The figure shows three views and two pictorial views of one solid part (mm, origin at its lowest corner). Answer the questions. Give positions to 0.01 mm unless a question says otherwise; leave off trailing zeros. Write each loop counter-clockwise with the first axis right and the second up, starting at its lowest first coordinate (ties: lowest second). Pieces come first, ordered by that corner, then holes. Notation, with made-up numbers: (-28, 89.5) - (14, 89.5) arc R8 ccw to (14, 104.5) - close; hole circle Ø8 at (76.5, -20.75). An arc over 180 degrees is marked (long way). Answer as CSV lines item,"result". Start each with the question number.
(1) Find section C-C (x = 269). Write down the section's boundary in (y, z).
(2) Find section B-B (y = 28). Write down the section's boundary in (x, z).
(3) Straight lines are drawn through the part: probe 1 along X at (y, z) = (12, 369); probe 2 along Z at (x, y) = (543, 39). For each, find the intervals that lie inside material, in ascending order.
(4) Find section A-A (z = 620.5). Write down the section's boundary in (x, y).
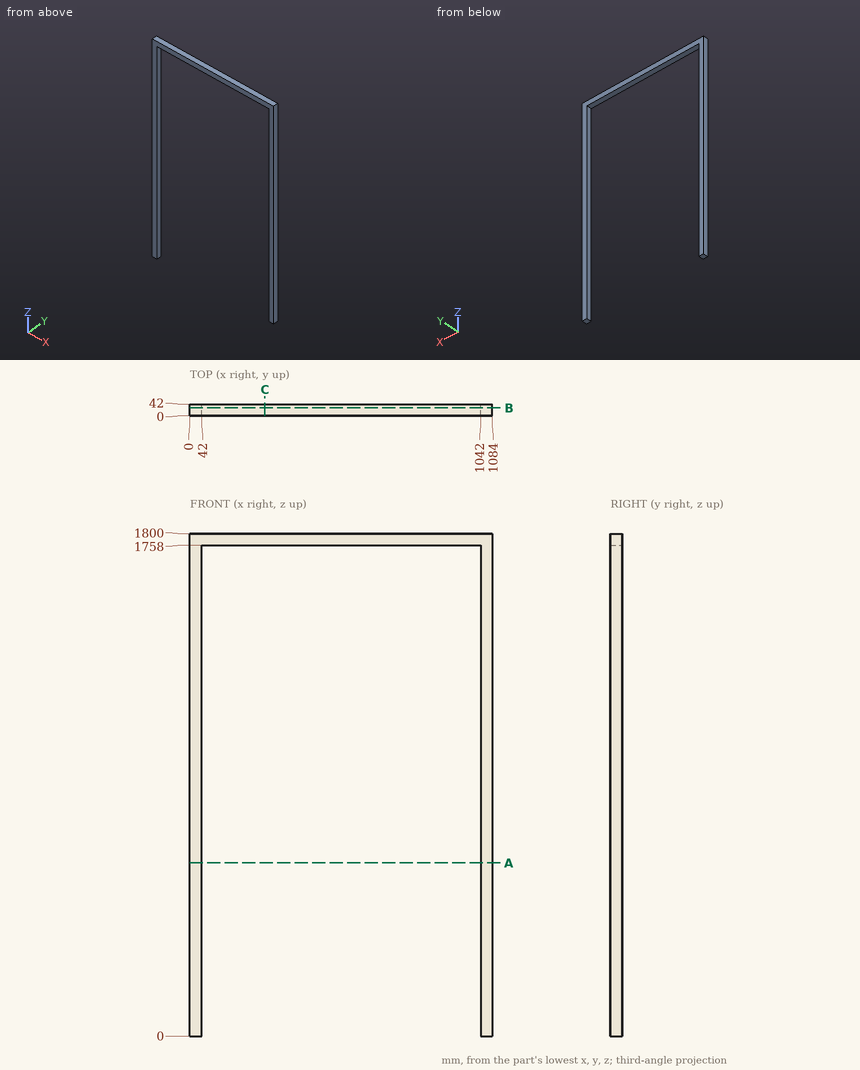
Result set:
1,outline,"(0, 1758) - (42, 1758) - (42, 1800) - (0, 1800) - close"
2,outline,"(0, 0) - (42, 0) - (42, 1758) - (1042, 1758) - (1042, 0) - (1084, 0) - (1084, 1800) - (0, 1800) - close"
3,probe 1,"0 to 42, 1042 to 1084"
3,probe 2,"1758 to 1800"
4,outline,"(0, 0) - (42, 0) - (42, 42) - (0, 42) - close; (1042, 0) - (1084, 0) - (1084, 42) - (1042, 42) - close"
